```python
from build123d import *

# Parameters (mm, degrees)
SKETCH1_R           = 20
BOSS_EXTRUDE1_DEPTH = 12
CUT_EXTRUDE1_DEPTH  = 6
BOSS_EXTRUDE2_DEPTH = 12
CIRPATTERN2_COUNT   = 10


with BuildPart() as part:
    # Sketch1 → Boss-Extrude1 (new body)
    with BuildSketch(Plane(origin=(0, 0, 0), x_dir=(1, 0, 0), z_dir=(0, 1, 0))):
        Circle(SKETCH1_R)
    extrude(amount=BOSS_EXTRUDE1_DEPTH)

    # Sketch2 → Cut-Extrude1 (cut)
    with BuildSketch(Plane(origin=(0, 12, 0), x_dir=(1, 0, 0), z_dir=(0, 1, 0))):
        with BuildLine():
            Line((-1.960372744, 1.614176032), (2.039627256, 1.614176032))
            ThreePointArc((2.039627256, 1.614176032), (2.539627256, 0.114176032), (2.039627256, -1.385823968))
            Line((2.039627256, -1.385823968), (-1.960372744, -1.385823968))
            ThreePointArc((-1.960372744, -1.385823968), (-2.460372744, 0.114176032), (-1.960372744, 1.614176032))
        make_face()
    extrude(amount=-CUT_EXTRUDE1_DEPTH, mode=Mode.SUBTRACT)

    # Sketch4 → Boss-Extrude2 (add)
    with BuildSketch(Plane(origin=(0, 12, 0), x_dir=(1, 0, 0), z_dir=(0, 1, 0))):
        with BuildLine():
            Line((-2.5, 30), (2.5, 30))
            ThreePointArc((2.5, 30), (4.041341884, 24.750944403), (5, 19.364916731))
            ThreePointArc((5, 19.364916731), (0, 20), (-5, 19.364916731))
            ThreePointArc((-5, 19.364916731), (-4.041341884, 24.750944403), (-2.5, 30))
        make_face()
    boss_extrude2 = extrude(amount=-BOSS_EXTRUDE2_DEPTH)

    # CirPattern2: Boss-Extrude2 ×10 about axis
    cirpattern2_axis = Axis((0, 0, 0), (0, 1, 0))
    for i in range(1, CIRPATTERN2_COUNT):
        add(boss_extrude2.rotate(cirpattern2_axis, i * 360 / CIRPATTERN2_COUNT))


solid = part.part
```
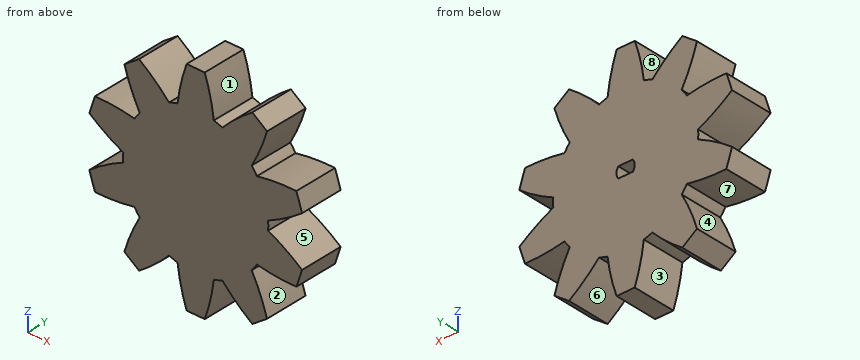
Geometry: final body of the model. Coordinates: model frame, mm. Face numbers are marked on the shaded views. A direction names the side the tool comes from. Round coordinates to 2 decimals unless told otherwise and drop trailing zeros. Loops run counter-clockwise (first coordinate to the right, second up) from the corner with the lowest first, then second, coordinate; pieces in that order, holes last.
Item 1: Section A-A, the plane x = -23. Output: boundary loops of the cut face in (y, z).
Checked values:
outline: (0, -11.55) - (12, -11.55) - (12, -2.77) - (0, -2.77) - close; (0, 2.77) - (12, 2.77) - (12, 11.55) - (0, 11.55) - close
Item 2: Section B-B, the plane z = -23.5. Output: boundary loops of the cut face in (x, y).
Checked values:
outline: (-18.69, 0) - (-12.6, 0) - (-12.6, 12) - (-18.69, 12) - close; (-4.32, 0) - (4.32, 0) - (4.32, 12) - (-4.32, 12) - close; (12.6, 0) - (18.69, 0) - (18.69, 12) - (12.6, 12) - close
Item 3: Line query: L1, parallel to X at y = 4, z = 25; L2, parallel to Z at x = 26, y = 0.75; L3, parallel to X at y = 9, z = -20. Output: solid intervals per line, ascending.
Checked values:
L1: x = -16.63 to -14.56, -3.98 to 3.98, 14.56 to 16.63
L2: z = -11.66 to -4.56, 4.56 to 11.66
L3: x = -18.74 to -8.69, -4.92 to 4.92, 8.69 to 18.74
Item 4: Section C-C, the plane z = 5. Output: boundary loops of the cut face in (x, y).
Checked values:
outline: (-26.66, 0) - (26.66, 0) - (26.66, 12) - (-26.66, 12) - close
Item 5: Reachability of the marked faces 4, 5, 6, 7 and 8 from +Z, -Z, +X, -X, +Y, -Y: full face, straight path, thin tool, end or side. Return the list, or none.
Checked values:
face 4: -X, +Y, -Y
face 5: +X, +Y, -Y
face 6: -Z, +Y, -Y
face 7: +Y, -Y
face 8: +Z, +Y, -Y
Item 6: Contact query for flat-ended pins moving along their axis: P1, Ø6, axis at y = 6.5, z = -1, coming from the -X side; P2, Ø4, axis at y = 6.5, z = -10, coming from the +X side; P3, Ø1, axis at x = 16, y = 7, coming from the -Z side. Output: stop coordinate, or through.
Checked values:
P1: stops at x = -25.11
P2: stops at x = 28.94
P3: stops at z = -25.74
Item 7: Mould query, pull axis Z, two halves, no side actions, for the marked faces 1, 2 and 3. Classes: released by +Z, released by -Z, zero draft, split by the parting line, or undercut.
Checked values:
face 1: released by +Z
face 2: undercut
face 3: released by -Z
Item 8: Section D-D, the plane x = 25. Output: boundary loops of the cut face in (y, z).
Checked values:
outline: (0, -11.64) - (12, -11.64) - (12, -3.93) - (0, -3.93) - close; (0, 3.93) - (12, 3.93) - (12, 11.64) - (0, 11.64) - close
